Verification items for the finished model (mm, model axes). A direction names the side the tool comes from. Round coordinates to 2 decimals unless told otherwise and drop trailing zeros. Loops run counter-clockwise (first coordinate to the right, second up) from the corner with the lowest first, then second, coordinate; pieces in that order, holes last.
from build123d import *

# Parameters (mm, degrees)
F0_W     = 25
F0_H     = 25
F1_DEPTH = 30
F2_R     = 1.25
F3_DEPTH = 60
F2_W     = 15
F2_H     = 15
F4_DEPTH = 0.5


with BuildPart() as f1:
    # F0 (on Top) → F1 (new body)
    with BuildSketch(Plane.XY):
        Rectangle(F0_W, F0_H)
    extrude(amount=F1_DEPTH)

    # F2 (on face) → F3 (join)
    with BuildSketch(Plane.XY.offset(30)):
        with Locations((-5, 5)):
            Circle(F2_R)
        with Locations((5, 5)):
            Circle(F2_R)
        with Locations((-5, -5)):
            Circle(F2_R)
        with Locations((5, -5)):
            Circle(F2_R)
    extrude(amount=F3_DEPTH)

    # F2 (on face) → F4 (join)
    with BuildSketch(Plane.XY.offset(30)):
        Rectangle(F2_W, F2_H)
        with Locations((-5, -5)):
            Circle(F2_R, mode=Mode.SUBTRACT)
        with Locations((5, -5)):
            Circle(F2_R, mode=Mode.SUBTRACT)
        with Locations((-5, 5)):
            Circle(F2_R, mode=Mode.SUBTRACT)
        with Locations((5, 5)):
            Circle(F2_R, mode=Mode.SUBTRACT)
    extrude(amount=F4_DEPTH)


solid = f1.part
1. Gauge pin test, flat ends, axial feed: P1, Ø5, axis at x = -8.5, y = 5.5, coming from the -Z side; P2, Ø2, axis at y = -8.5, z = 37.5, coming from the +X side; P3, Ø4, axis at x = 4, z = 35, coming from the -Y side; P4, Ø1.5, axis at x = 3.5, z = 71, coming from the +Y side. Record the tip position at first contact, or that the pin passes through.
2. Release check for a two-part mould opening along Y. For faces 3 (the face through (0, 0, 0)), 4 (the face through (0, 12.5, 15)), 5 (the face through (0, -12.5, 15)), 6 (the face through (-5.27, -6.22, 59.83)) record: released by +Y, released by -Y, zero draft, split by the parting line, or undercut.
3. Section check C-C (z = 41.5). Enter the section's corners in (x, y), then the cut area to 3 significant figures.
4. Section check A-A (x = 5). Enter the section's corners in (y, z).
5. Scan lines: L1, parallel to Z at x = -3, y = -7.75; L2, parallel to Z at x = 1.75, y = -3; L3, parallel to Y at x = -5, z = 84. Record each from-to range of solid material in increasing order.
6. Section check D-D (y = -0.75). Enter the section's corners in (x, z).
7. Tool access check on faces 1 (the face through (-5.27, 3.78, 59.83)), 2 (the face through (5, 5, 90)). Record the directions out of +Z, -Z, +X, -X, +Y, -Y that give a thin tool (end or side, any length) a straight path to the whole face; none if there is none.
Taken from the geometry:
1. P1: stops at z = 0
1. P2: passes through
1. P3: stops at y = -6.25
1. P4: stops at y = 6
2. face 3: zero draft
2. face 4: released by +Y
2. face 5: released by -Y
2. face 6: undercut
3. outline: circle Ø2.5 at (-5, -5); circle Ø2.5 at (-5, 5); circle Ø2.5 at (5, -5); circle Ø2.5 at (5, 5)
3. area: 19.6 mm2
4. outline: (-12.5, 0) - (12.5, 0) - (12.5, 30) - (7.5, 30) - (7.5, 30.5) - (6.25, 30.5) - (6.25, 90) - (3.75, 90) - (3.75, 30.5) - (-3.75, 30.5) - (-3.75, 90) - (-6.25, 90) - (-6.25, 30.5) - (-7.5, 30.5) - (-7.5, 30) - (-12.5, 30) - close
5. L1: z = 0 to 30
5. L2: z = 0 to 30.5
5. L3: y = -6.25 to -3.75, 3.75 to 6.25
6. outline: (-12.5, 0) - (12.5, 0) - (12.5, 30) - (7.5, 30) - (7.5, 30.5) - (-7.5, 30.5) - (-7.5, 30) - (-12.5, 30) - close
7. face 1: +Z
7. face 2: +Z, +X, -X, +Y, -Y
